from build123d import *

# Parameters (mm, degrees)
SALIENTE_EXTRUIR2_DEPTH = 3
SALIENTE_EXTRUIR3_DEPTH = 70
CROQUIS_HUECO_MOTOR_W   = 23
CROQUIS_HUECO_MOTOR_H   = 67
HUECO_MOTOR_DEPTH       = 5
CROQUIS10_R             = 2.4
CROQUIS10_R_2           = 2
TORNILLO_Y_MOTOR_DEPTH  = 5
CROQUIS12_W             = 23
CROQUIS12_H             = 5
SALIENTE_EXTRUIR5_DEPTH = 4
CROQUIS16_R             = 2
CORTAR_EXTRUIR4_DEPTH   = 77.893188905


with BuildPart() as part:
    # Croquis4 → Saliente-Extruir2 (new body)
    with BuildSketch(Plane.XY):
        Polygon((14.5, 16), (-14.5, 16), (-14.5, 8), (-24.75, 8), (-24.75, -7), (-14.5, -7), (-14.5, -15), (14.5, -15), (14.5, -7), (24.75, -7), (24.75, 8), (14.5, 8), align=None)
    extrude(amount=SALIENTE_EXTRUIR2_DEPTH)

    # Croquis5 → Saliente-Extruir3 (add)
    with BuildSketch(Plane(origin=(0, 0, 0), x_dir=(-1, 0, 0), z_dir=(0, 0, -1))):
        Polygon((-24.75, -4), (-24.75, -7), (-14.5, -7), (-14.5, -15), (14.5, -15), (14.5, -7), (24.75, -7), (24.75, -4), align=None)
    extrude(amount=SALIENTE_EXTRUIR3_DEPTH)

    # croquis hueco motor → hueco motor (cut)
    with BuildSketch(Plane(origin=(0, -4, 0), x_dir=(1, 0, 0), z_dir=(0, 1, 0))):
        with Locations((0, 33.5)):
            Rectangle(CROQUIS_HUECO_MOTOR_W, CROQUIS_HUECO_MOTOR_H)
    extrude(amount=-HUECO_MOTOR_DEPTH, mode=Mode.SUBTRACT)

    # Croquis10 → tornillo y motor (cut)
    with BuildSketch(Plane.XY.offset(3)):
        with Locations((0, 0.5)):
            Circle(CROQUIS10_R)
        with Locations((-18.6, 0.5)):
            Circle(CROQUIS10_R_2)
        with Locations(Location((18.6, 0.5, 0), (0, 0, 180))):
            Circle(CROQUIS10_R_2)
    extrude(amount=-TORNILLO_Y_MOTOR_DEPTH, mode=Mode.SUBTRACT)

    # Croquis12 → Saliente-Extruir5 (add)
    with BuildSketch(Plane(origin=(0, -9, 0), x_dir=(1, 0, 0), z_dir=(0, 1, 0))):
        with Locations((0, 64.5)):
            Rectangle(CROQUIS12_W, CROQUIS12_H)
    extrude(amount=SALIENTE_EXTRUIR5_DEPTH)

    # Croquis16 → Cortar-Extruir4 (cut, through all)
    with BuildSketch(Plane(origin=(0, -4, 0), x_dir=(1, 0, 0), z_dir=(0, 1, 0))):
        with Locations(Location((-18.63, 52.5, 0), (0, 0, 180))):
            Circle(CROQUIS16_R)
        with Locations(Location((-18.63, 14.5, 0), (0, 0, 270))):
            Circle(CROQUIS16_R)
        with Locations(Location((18.63, 14.5, 0), (0, 0, 180))):
            Circle(CROQUIS16_R)
        with Locations(Location((18.63, 52.5, 0), (0, 0, 180))):
            Circle(CROQUIS16_R)
    extrude(amount=-CORTAR_EXTRUIR4_DEPTH, mode=Mode.SUBTRACT)


solid = part.part
Model file for the job. Use its own axes, mm. A direction names the side the tool comes from. Coordinates: 2 decimals unless noted, no trailing zeros. Write each loop counter-clockwise with the first axis right and the second up, starting at its lowest first coordinate (ties: lowest second). Pieces come first, ordered by that corner, then holes. Notation, with made-up numbers: (32, 48.25) -> (56, 48.25) arc R30 cw to (56, 77.25) -> close; hole circle Ø5 at (82.25, 74.5). An arc over 180 degrees is marked (long way). One line per item, written item: value. Start each with the question number.
1) Which spindle directions (+Z, -Z, +X, -X, +Y, -Y) get a long thin tool onto all of the face, cutting with end or side? Do faces 3 (the face through (14.5, 12, 1)), 4 (the face through (14.5, -11, -33)), 5 (the face through (-14.5, 12, 1)), 6 (the face through (-11.5, -6, -33)), 7 (the face through (16, -4, -35)). Say none if no direction does.
2) Slice it at A-A on z = -52.5. Write the cut outline in (x, y).
3) Probe probe 1 along Y at (x, z) = (-18.6, 1.75); probe 2 along X at (y, z) = (0, 1); probe 3 along Z at (x, y) = (-18, -6). List the from-to ranges inside material, lowest first.
4) Slice it at C-C on y = 0.5. Write the cut outline in (x, z).
5) Flat gauge pins, fed straight in: pin 1 Ø3.5 at (x, z) = (19.5, 1.5) entering from +Y; pin 2 Ø1.5 at (y, z) = (12, 1.5) entering from -X; pin 3 Ø11.5 at (x, z) = (-22, -25.5) entering from -Y; pin 4 Ø2.5 at (x, z) = (18.63, -14.5) entering from +Y. Where does each tip first touch, or does it go through?
6) Slice it at B-B on x = 0. Write the cut outline in (y, z).
7) Slice it at D-D on x = 18.63. Write the cut outline in (y, z).
8) Pull direction Z, two halves, no side cores. Call faces 1 (the face through (-20, -7, -33)), 2 (the face through (-19.553, -5.479, -54.274)): +Z half, -Z half, draft (parallel to the pull), parting line (faces both ways), or undercut.
Answers follow:
1. face 3: +Z, -Z, +X, +Y
1. face 4: +Z, -Z, +X, -Y
1. face 5: +Z, -Z, -X, +Y
1. face 6: +Y
1. face 7: -Z, +X, -X, +Y
2. outline: (-24.75, -7) -> (-20.63, -7) -> (-20.63, -4) -> (-24.75, -4) -> close; (-16.63, -7) -> (-14.5, -7) -> (-14.5, -15) -> (14.5, -15) -> (14.5, -7) -> (16.63, -7) -> (16.63, -4) -> (11.5, -4) -> (11.5, -9) -> (-11.5, -9) -> (-11.5, -4) -> (-16.63, -4) -> close; (20.63, -7) -> (24.75, -7) -> (24.75, -4) -> (20.63, -4) -> close
3. probe 1: -7 to -1.5, 2.5 to 8
3. probe 2: -24.75 to -20.54, -16.66 to -2.35, 2.35 to 16.66, 20.54 to 24.75
3. probe 3: -70 to -54.4, -50.6 to -16.4, -12.6 to 3
4. outline: (-24.75, 0) -> (-20.6, 0) -> (-20.6, 3) -> (-24.75, 3) -> close; (-16.6, 0) -> (-2.4, 0) -> (-2.4, 3) -> (-16.6, 3) -> close; (2.4, 0) -> (16.6, 0) -> (16.6, 3) -> (2.4, 3) -> close; (20.6, 0) -> (24.75, 0) -> (24.75, 3) -> (20.6, 3) -> close
5. pin 1: y = 8
5. pin 2: x = -14.5
5. pin 3: y = -7
5. pin 4: through
6. outline: (-15, -70) -> (-4, -70) -> (-4, -67) -> (-5, -67) -> (-5, -62) -> (-9, -62) -> (-9, 0) -> (-1.9, 0) -> (-1.9, 3) -> (-15, 3) -> close; (2.9, 0) -> (16, 0) -> (16, 3) -> (2.9, 3) -> close
7. outline: (-7, -70) -> (-4, -70) -> (-4, -54.5) -> (-7, -54.5) -> close; (-7, -50.5) -> (-4, -50.5) -> (-4, -16.5) -> (-7, -16.5) -> close; (-7, -12.5) -> (-4, -12.5) -> (-4, 0) -> (-1.5, 0) -> (-1.5, 3) -> (-7, 3) -> close; (2.5, 0) -> (8, 0) -> (8, 3) -> (2.5, 3) -> close
8. face 1: draft
8. face 2: undercut
